```python
from build123d import *

# Parameters (mm, degrees)
F0_W     = 2530
F0_H     = 1150
F1_DEPTH = 28.9
F2_W     = 2504
F2_H     = 1124
F3_DEPTH = 28.1
F4_W     = 2528.4
F4_H     = 1148.4
F5_DEPTH = 27.3


with BuildPart() as f1:
    # F0 (on Front) → F1 (new body)
    with BuildSketch(Plane.XZ):
        with Locations((1265, 575)):
            Rectangle(F0_W, F0_H)
    extrude(amount=F1_DEPTH)

    # F2 (on face) → F3 (cut)
    with BuildSketch(Plane.XZ.offset(28.9)):
        with Locations((1265, 575)):
            Rectangle(F2_W, F2_H)
    extrude(amount=-F3_DEPTH, mode=Mode.SUBTRACT)

    # F4 (on face) → F5 (cut)
    with BuildSketch(Plane.XZ.offset(0.8)):
        with Locations((1265, 575)):
            Rectangle(F4_W, F4_H)
    extrude(amount=F5_DEPTH, mode=Mode.SUBTRACT)


solid = f1.part
```
Can you work these out from the model? Positions are in its coordinate system, mm. Give positions to 0.01 mm unless a question says otherwise; leave off trailing zeros. Write each loop counter-clockwise with the first axis right and the second up, starting at its lowest first coordinate (ties: lowest second). Pieces come first, ordered by that corner, then holes. Notation, with made-up numbers: (-17, -12.5) -> (1, -12.5) arc R8 ccw to (1, -1.5) -> close; hole circle Ø7 at (5, -21). An arc over 180 degrees is marked (long way). One line per item, written item: value.
Q1. Imagine slicing it at B-B on x = 2179.5. Please give me the cut outline in (y, z).
Results found:
outline: (-28.9, 0) -> (0, 0) -> (0, 1150) -> (-28.9, 1150) -> (-28.9, 1137) -> (-28.1, 1137) -> (-28.1, 1149.2) -> (-0.8, 1149.2) -> (-0.8, 0.8) -> (-28.1, 0.8) -> (-28.1, 13) -> (-28.9, 13) -> close
Q2. Imagine slicing it at C-C on z = 693.5. Please give me the cut outline in (x, y).
Results found:
outline: (0, -28.9) -> (13, -28.9) -> (13, -28.1) -> (0.8, -28.1) -> (0.8, -0.8) -> (2529.2, -0.8) -> (2529.2, -28.1) -> (2517, -28.1) -> (2517, -28.9) -> (2530, -28.9) -> (2530, 0) -> (0, 0) -> close
Q3. We'd pull the mould along Z, two halves only. Please class faces 1 (the face through (1247, -0.8, 583)), 2 (the face through (1247, 0, 583)): +Z half, -Z half, draft (parallel to the pull), parting line (faces both ways), or undercut.
Results found:
face 1: undercut
face 2: draft
Q4. For P1, Ø1.5, axis at x = 897, z = 401, coming from the -Y side; P2, Ø3, axis at y = -11, z = 641.5, coming from the -X side, each with a flat end and sliding along its axis, tell me the tip position at first contact or that it passes through.
Results found:
P1: stops at y = -0.8
P2: stops at x = 0
Q5. Imagine slicing it at A-A on y = -23.75. Please give me the cut outline in (x, z), and give its area (3 significant figures).
Results found:
outline: (0, 0) -> (2530, 0) -> (2530, 1150) -> (0, 1150) -> close; hole (0.8, 0.8) -> (2529.2, 0.8) -> (2529.2, 1149.2) -> (0.8, 1149.2) -> close
area: 5,890 mm^2
Q6. Please list where these lines run through material, in increasing order: line 1 (X direction, y = -12, z = 706); line 2 (Z direction, x = 116, y = -5); line 3 (Y direction, x = 705, z = 559). Write a range as [from, to].
Results found:
line 1: x = [0, 0.8], [2529.2, 2530]
line 2: z = [0, 0.8], [1149.2, 1150]
line 3: y = [-0.8, 0]
